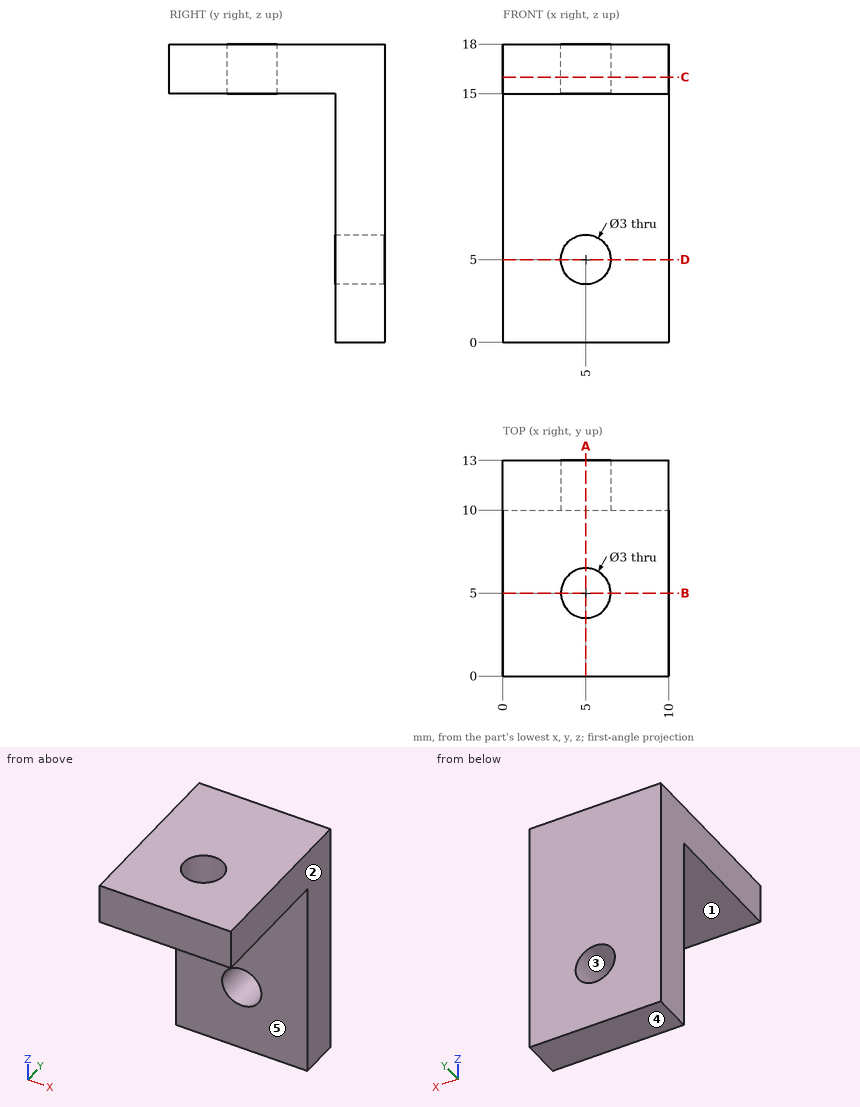
The figure shows three views and two pictorial views of one solid part (mm, origin at its lowest corner). Answer the questions. A direction names the side the tool comes from. Give positions to 0.01 mm unless a question says otherwise; leave off trailing zeros. Write each loop counter-clockwise with the first axis right and the second up, starting at its lowest first coordinate (ties: lowest second). Pieces come first, ordered by that corner, then holes. Notation, with made-up numbers: (53.25, 42.5) -> (112.25, 42.5) arc R27 ccw to (112.25, 70.5) -> close; hole circle Ø4 at (26, -5). An arc over 180 degrees is marked (long way). Use one line per item in the form item = value.
1) A tool of negligible diameter and unlimited length cuts with its end or side. For the marked faces 4 and 5, from which of +Z, -Z, +X, -X, +Y, -Y can it reach the whole face along a straight path? Write none if from no direction.
Result:
face_4 = -Z, +X, -X, +Y, -Y
face_5 = -Z, +X, -X, -Y
2) Section A-A on x = 5 is taken. Write down the section's boundary in (y, z), plus the area to 3 significant figures.
Result:
outline = (0, 15) -> (3.5, 15) -> (3.5, 18) -> (0, 18) -> close; (6.5, 15) -> (10, 15) -> (10, 6.5) -> (13, 6.5) -> (13, 18) -> (6.5, 18) -> close; (10, 0) -> (13, 0) -> (13, 3.5) -> (10, 3.5) -> close
area = 66.0 mm²
3) This flat-tipped pin is pushed along its axis until it touches: P1, Ø5, axis at x = 6.5, z = 9, coming from the -Y side. Where does it stop, or does it pass through?
Result:
P1 = 10
4) Section C-C on z = 16 is taken. Write down the section's boundary in (x, y).
Result:
outline = (0, 0) -> (10, 0) -> (10, 13) -> (0, 13) -> close; hole circle Ø3 at (5, 5)
5) Section B-B on y = 5 is taken. Write down the section's boundary in (x, z).
Result:
outline = (0, 15) -> (3.5, 15) -> (3.5, 18) -> (0, 18) -> close; (6.5, 15) -> (10, 15) -> (10, 18) -> (6.5, 18) -> close
6) For a pull along X with two mould halves and no side action, classify the marked faces 1, 2 and 3 as +X half, -X half, draft (parallel to the pull), parting line (faces both ways), or undercut.
Result:
face_1 = draft
face_2 = +X half
face_3 = undercut
7) Straight lines are drawn through the part: probe 1 along Y at (x, z) = (5, 17.3); probe 2 along Y at (x, z) = (2.5, 11); probe 3 along Z at (x, y) = (3, 6.25). For each, find the intervals that lie inside material, in ascending order.
Result:
probe_1 = 0 to 3.5, 6.5 to 13
probe_2 = 10 to 13
probe_3 = 15 to 18
8) Section D-D on z = 5 is taken. Write down the section's boundary in (x, y).
Result:
outline = (0, 10) -> (3.5, 10) -> (3.5, 13) -> (0, 13) -> close; (6.5, 10) -> (10, 10) -> (10, 13) -> (6.5, 13) -> close
